Verification items for this drawing (mm, ordinates from the low corner). A direction names the side the tool comes from. Round coordinates to 2 decimals unless told otherwise and drop trailing zeros. Loops run counter-clockwise (first coordinate to the right, second up) from the corner with the lowest first, then second, coordinate; pieces in that order, holes last. Notation, with made-up numbers: (9.25, 4) - (66.25, 4) arc R19 ccw to (66.25, 16) - close; hole circle Ø8 at (-32, 4). An arc over 180 degrees is marked (long way). Put each result on its own line as item: value.
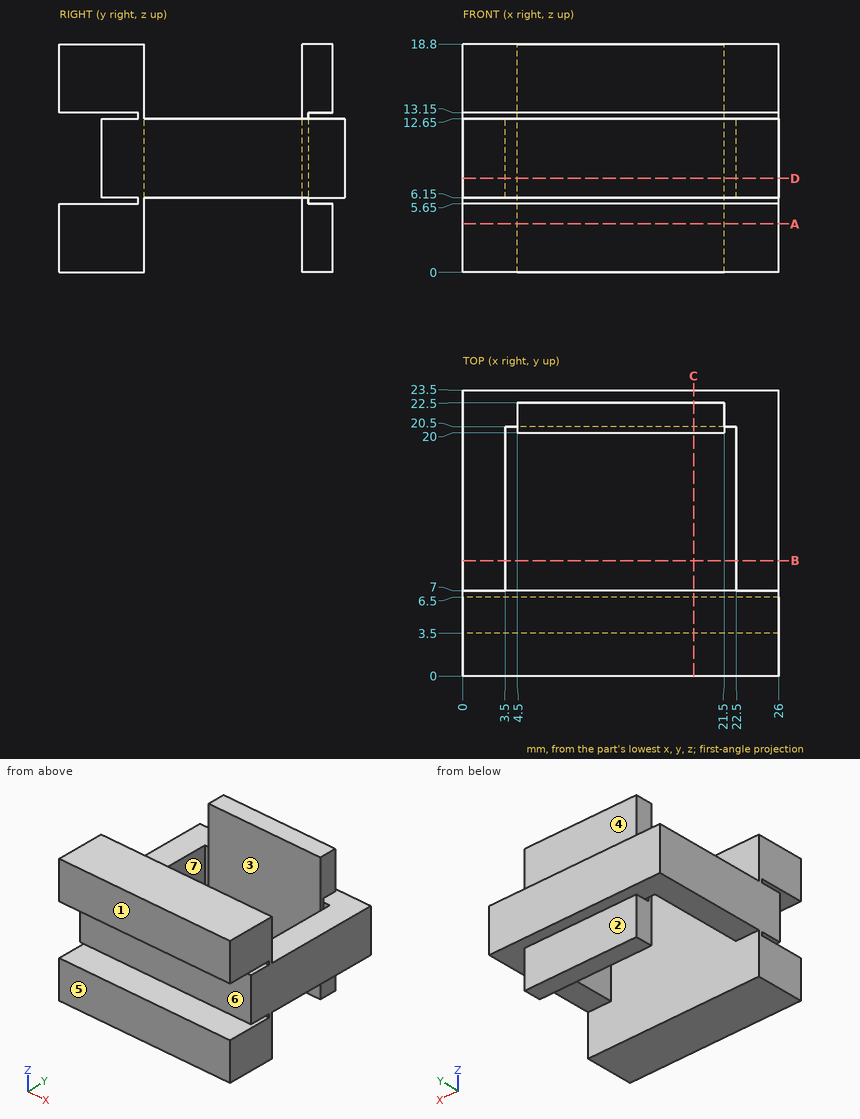
Item 1: Go/stop test with flat-tipped pins: pin 1 (1.1 mm diameter, centred on x = 4, z = 10, fed in from -Y); pin 2 (1 mm diameter, centred on y = 21, z = 2.5, fed in from +X); pin 3 (6 mm diameter, centred on x = 15.5, z = 1.5, fed in from +Y). Record where each tip stops, or that it passes through.
Filled sheet:
pin 1: y = 3.5
pin 2: x = 21.5
pin 3: y = 22.5
Item 2: Section check A-A on z = 4. Enter the section's corners in (x, y).
Filled sheet:
outline: (0, 0) - (26, 0) - (26, 7) - (0, 7) - close; (4.5, 20) - (21.5, 20) - (21.5, 22.5) - (4.5, 22.5) - close
Item 3: Thickness scan on line 1 (Y direction, x = 16.25, z = 10); line 2 (Z direction, x = 4.5, y = 1.5); line 3 (Y direction, x = 22.25, z = 8). Record the ranges inside material, lowest first. Write a range as from..to.
Filled sheet:
line 1: 3.5..7, 20..23.5
line 2: 0..5.65, 13.15..18.8
line 3: 3.5..7, 20.5..23.5
Item 4: Release check for a two-part mould opening along Y. For the marked faces 1, 2 and 3 record: +Y half, -Y half, draft (parallel to the pull), parting line (faces both ways), or undercut.
Filled sheet:
face 1: -Y half
face 2: +Y half
face 3: undercut
Item 5: Section check D-D on z = 7.75. Enter the section's corners in (x, y).
Filled sheet:
outline: (0, 3.5) - (26, 3.5) - (26, 23.5) - (0, 23.5) - close; hole (3.5, 7) - (22.5, 7) - (22.5, 20.5) - (21.5, 20.5) - (21.5, 20) - (4.5, 20) - (4.5, 20.5) - (3.5, 20.5) - close
Item 6: Section check C-C on x = 19. Enter the section's corners in (y, z), then the cut area to 3 significant figures.
Filled sheet:
outline: (0, 0) - (7, 0) - (7, 18.8) - (0, 18.8) - (0, 13.15) - (6.5, 13.15) - (6.5, 12.65) - (3.5, 12.65) - (3.5, 6.15) - (6.5, 6.15) - (6.5, 5.65) - (0, 5.65) - close; (20, 0) - (22.5, 0) - (22.5, 5.65) - (20.5, 5.65) - (20.5, 6.15) - (23.5, 6.15) - (23.5, 12.65) - (20.5, 12.65) - (20.5, 13.15) - (22.5, 13.15) - (22.5, 18.8) - (20, 18.8) - close
area: 154 mm²
Item 7: Tool access check on the marked faces 4, 5, 6 and 7. Record the directions out of +Z, -Z, +X, -X, +Y, -Y that give a thin tool (end or side, any length) a straight path to the whole face; none if there is none.
Filled sheet:
face 4: +Z, +X, -X, +Y
face 5: +Z, -Z, +X, -X, -Y
face 6: +X, -X, -Y
face 7: +Z, -Z
Item 8: Section check B-B on y = 9.5. Enter the section's corners in (x, z), then the cut area to 3 significant figures.
Filled sheet:
outline: (0, 6.15) - (3.5, 6.15) - (3.5, 12.65) - (0, 12.65) - close; (22.5, 6.15) - (26, 6.15) - (26, 12.65) - (22.5, 12.65) - close
area: 45.5 mm²
